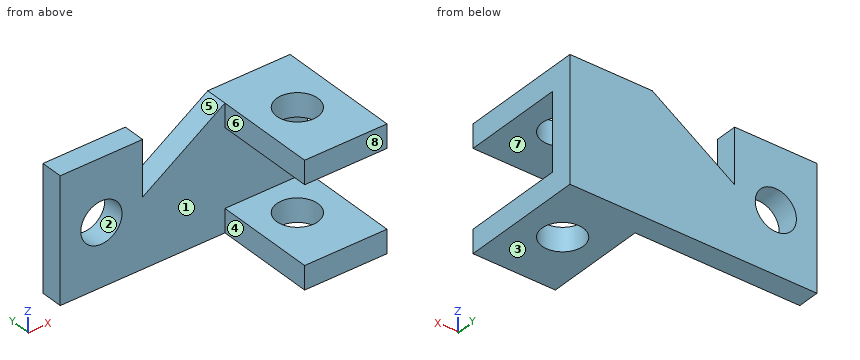
from build123d import *

# Parameters (mm, degrees)
F1_DEPTH = 8
F2_W     = 30
F2_H     = 8.5
F3_DEPTH = 37
F4_R     = 7.5
F5_DEPTH = 45.001
F6_R     = 7.5
F7_DEPTH = 8.001


with BuildPart() as f1:
    # F0 (on Front) → F1 (new body)
    with BuildSketch(Plane.XZ):
        Polygon((-41.746499, -28.969837), (48.253501, -28.969837), (48.253501, 16.030163), (18.253501, 16.030163), (-11.746499, -3.969837), (-11.746499, 16.030163), (-41.746499, 16.030163), align=None)
    extrude(amount=F1_DEPTH)

    # F2 (on face) → F3 (join)
    with BuildSketch(Plane.XZ.offset(8)):
        with Locations((33.253501, 11.780163)):
            Rectangle(F2_W, F2_H)
        with Locations((33.253501, -24.719837)):
            Rectangle(F2_W, F2_H)
    extrude(amount=F3_DEPTH)

    # F4 (on face) → F5 (cut, through all)
    with BuildSketch(Plane.XY.offset(16.030163)):
        with Locations((33.253501, -22.5)):
            Circle(F4_R)
    extrude(amount=-F5_DEPTH, mode=Mode.SUBTRACT)

    # F6 (on face) → F7 (cut, through all)
    with BuildSketch(Plane.XZ.offset(8)):
        with Locations((-26.746499, -6.469837)):
            Circle(F6_R)
    extrude(amount=-F7_DEPTH, mode=Mode.SUBTRACT)


solid = f1.part
Can you work these out from the model? Positions are in its coordinate system, mm. Face numbers are marked on the shaded views. A direction names the side the tool comes from. Round coordinates to 2 decimals unless told otherwise and drop trailing zeros. Write each loop counter-clockwise with the first axis right and the second up, starting at its lowest first coordinate (ties: lowest second). Pieces come first, ordered by that corner, then holes. Notation, with made-up numbers: M -16,-18 L -4,-18 A9 ccw -4,-14 Z; hole C 51,73.25 d8. An arc over 180 degrees is marked long. Use a Markdown table: item, result.
Item 1: I want a section at B-B (z = 9). List the corners of the cut face in (x, y) for me, and give its area (3 significant figures).
Found:
| item | result |
|---|---|
| outline | M -41.75,-8 L -11.75,-8 L -11.75,0 L -41.75,0 Z; M 7.71,-8 L 18.25,-8 L 18.25,-45 L 48.25,-45 L 48.25,0 L 7.71,0 Z; hole C 33.25,-22.5 d15 |
| area | 1,500 mm2 |
Item 2: I want a section at A-A (y = -38). List the corners of the cut face in (x, z) for me.
Found:
| item | result |
|---|---|
| outline | M 18.25,-28.97 L 48.25,-28.97 L 48.25,-20.47 L 18.25,-20.47 Z; M 18.25,7.53 L 48.25,7.53 L 48.25,16.03 L 18.25,16.03 Z |
Item 3: If I drill on line 1 along Z through (x, y) = (37, -9); line 2 along X through (y, z) = (-22, -25); line 3 along X through (y, z) = (-13.5, 10.5), over which ranges is the centre line in solid material (lowest first)? Write a range as [from, to].
Found:
| item | result |
|---|---|
| line 1 | z = [-28.97, -20.47], [7.53, 16.03] |
| line 2 | x = [18.25, 25.77], [40.74, 48.25] |
| line 3 | x = [18.25, 48.25] |
Item 4: For pin 1 Ø5 at (x, z) = (-32, -20) entering from -Y; pin 2 Ø2.5 at (y, z) = (-30.5, -25.5) entering from -X, each with a flat end and sliding along its axis, tell me the tip position at first contact or that it passes through.
Found:
| item | result |
|---|---|
| pin 1 | stops at y = -8 |
| pin 2 | stops at x = 18.25 |
Item 5: Which directions (+Z, -Z, +X, -X, +Y, -Y) give clear straight access to the entire face, cutting with the end or side of a thin tool? Please do the marked faces 5, 6, 7 and 8.
Found:
| item | result |
|---|---|
| face 5 | +Z, +Y, -Y |
| face 6 | +Z, -Z, -X, -Y |
| face 7 | +X, -X, -Y |
| face 8 | +Z, -Z, +X, -X, -Y |
Item 6: We'd pull the mould along Z, two halves only. Please class the marked faces 1, 2, 3 and 4: released by +Z, released by -Z, zero draft, split by the parting line, or undercut.
Found:
| item | result |
|---|---|
| face 1 | undercut |
| face 2 | undercut |
| face 3 | released by -Z |
| face 4 | zero draft |
Item 7: I want a section at D-D (y = -22.5). List the corners of the cut face in (x, z) for me, and give its area (3 significant figures).
Found:
| item | result |
|---|---|
| outline | M 18.25,-28.97 L 25.75,-28.97 L 25.75,-20.47 L 18.25,-20.47 Z; M 18.25,7.53 L 25.75,7.53 L 25.75,16.03 L 18.25,16.03 Z; M 40.75,-28.97 L 48.25,-28.97 L 48.25,-20.47 L 40.75,-20.47 Z; M 40.75,7.53 L 48.25,7.53 L 48.25,16.03 L 40.75,16.03 Z |
| area | 255 mm2 |
Item 8: I want a section at C-C (z = -23.5). List the corners of the cut face in (x, y) for me, and give its area (3 significant figures).
Found:
| item | result |
|---|---|
| outline | M -41.75,-8 L 18.25,-8 L 18.25,-45 L 48.25,-45 L 48.25,0 L -41.75,0 Z; hole C 33.25,-22.5 d15 |
| area | 1,650 mm2 |
